Job drawing, mm, ordinate dimensions from the low corner. One solid piece. Give positions to 0.01 mm unless a question says otherwise; leave off trailing zeros. Order: outer loops, then holes, each group sorted by start corner. A loop starts at its lowest first (then second) coordinate and runs counter-clockwise, first axis right, second up. Notation, with made-up numbers: (-6, 67.25) -> (41, 67.25) arc R27 cw to (41, 99.25) -> close; hole circle Ø3 at (37.25, 55). An arc over 180 degrees is marked (long way). Use CSV: the item, a comma, the result in double quotes. Start each with the question number.
1. Cut at B-B on y = 12.75. List the corners of the cut face in (x, z) (1 decimal).
2. Cut at A-A on z = 52.5. List the corners of the cut face in (x, y) (1 decimal), then the cut area to 3 significant figures.
3. Pull direction Z, two halves, no side cores. Call the marked faces 1 and 2: released by +Z, released by -Z, zero draft, split by the parting line, or undercut.
4. Cut at C-C on x = 26.5. List the corners of the cut face in (y, z) (1 decimal).
5. Wall check: line 1 (Y direction, x = 49, z = 39); line 2 (X direction, y = 11.75, z = 65.5) (1 decimal). Give the ranges that are in metal, low to high. Write a range as from..to.
6. Drop flat-ended pins along their axis: pin 1 (2 mm diameter, centred on y = 11, z = 74, fed in from -X); pin 2 (3 mm diameter, centred on x = 16, z = 25, fed in from +Y); pin 3 (2 mm diameter, centred on y = 11.5, z = 71.5, fed in from +X) (1 decimal). Give the stop position or say it passes through.
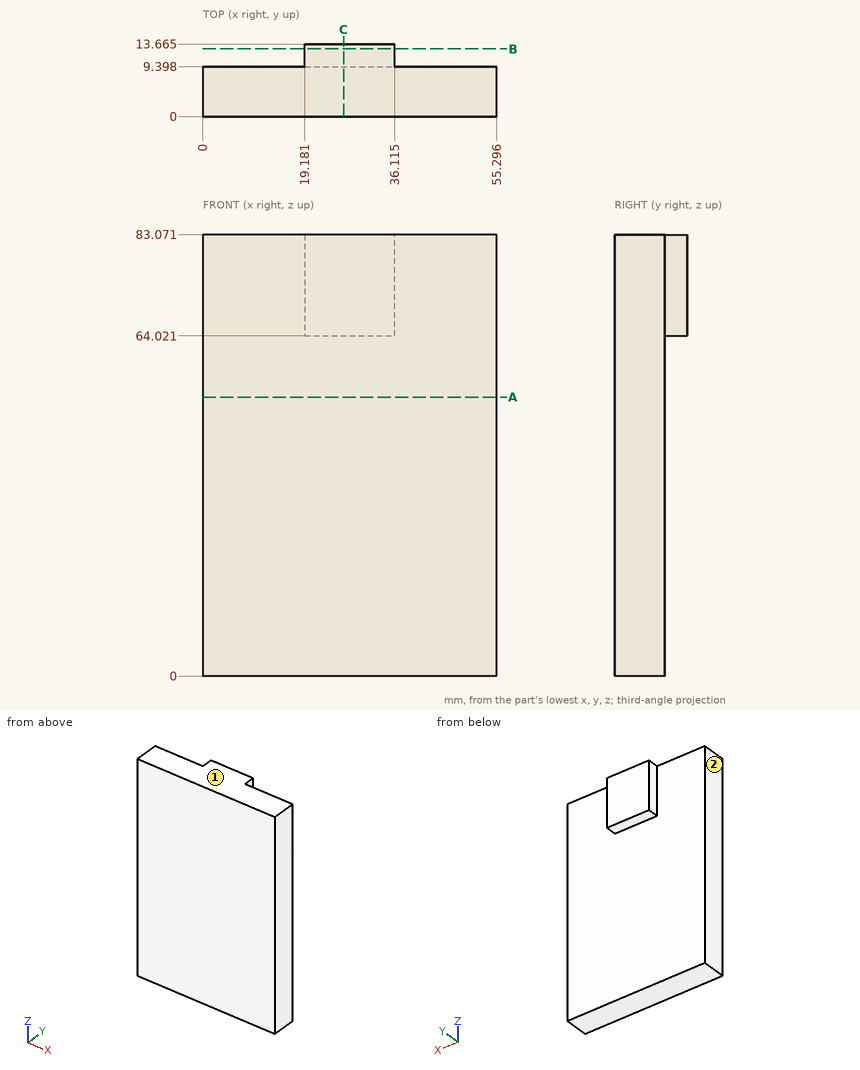
Verdict:
1,outline,"(19.2, 64) -> (36.1, 64) -> (36.1, 83.1) -> (19.2, 83.1) -> close"
2,outline,"(0, 0) -> (55.3, 0) -> (55.3, 9.4) -> (0, 9.4) -> close"
2,area,"520 mm^2"
3,face 1,"released by +Z"
3,face 2,"zero draft"
4,outline,"(0, 0) -> (9.4, 0) -> (9.4, 64) -> (13.7, 64) -> (13.7, 83.1) -> (0, 83.1) -> close"
5,line 1,"0..9.4"
5,line 2,"19.2..36.1"
6,pin 1,"x = 19.18"
6,pin 2,"y = 9.4"
6,pin 3,"x = 36.1"
